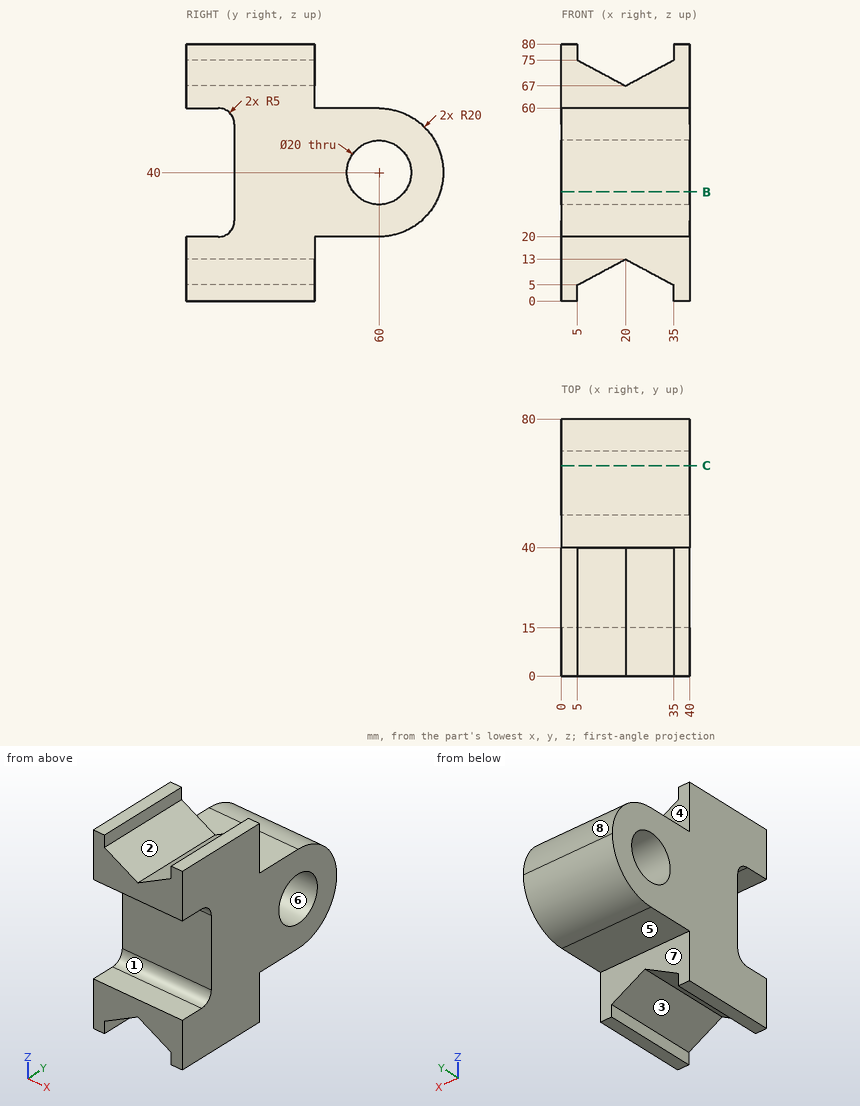
Input: dimensioned drawing with shaded views. Units: mm. Origin: part minimum x, y, z. A direction names the side the tool comes from. Round coordinates to 2 decimals unless told otherwise and drop trailing zeros. Order: outer loops, then holes, each group sorted by start corner. A loop starts at its lowest first (then second) coordinate and runs counter-clockwise, first axis right, second up. Notation, with made-up numbers: (73, 35.25) -> (102, 35.25) arc R15 cw to (102, 42.25) -> close; hole circle Ø2 at (-9, -13.5). An arc over 180 degrees is marked (long way). Put each result on its own line as item: value. Start each with the question number.
Q1. Section C-C on y = 65.5. Return the cut outline in (x, z).
Q2. First-contact query: pin 1 (6 mm diameter, centred on x = 12.5, y = 50.5, fed in from +Z); pin 2 (10 mm diameter, centred on x = 11, z = 70, fed in from +Y); pin 3 (22 mm diameter, centred on x = 16.5, z = 12, fed in from +Y). Flat tips, straight axial feed; report the tip coordinate or a pass-through.
Q3. Line query: probe 1 along Z at (x, y) = (13, 60); probe 2 along Y at (x, z) = (10, 40); probe 3 along Z at (x, y) = (2, 8.5). Output: solid intervals per line, ascending.
Q4. Section B-B on z = 34. Return the cut outline in (x, y).
Q5. Reachability of the marked faces 1, 2, 3, 4 and 5 from +Z, -Z, +X, -X, +Y, -Y: full face, straight path, thin tool, end or side. Return the list, or none.
Q6. Pull-direction query (Z, two-part tool) for the marked faces 6, 7 and 8; classes: +Z half, -Z half, draft (parallel to the pull), parting line (faces both ways), or undercut.
Ans:
1. outline: (0, 20.77) -> (40, 20.77) -> (40, 31.65) -> (0, 31.65) -> close; (0, 48.35) -> (40, 48.35) -> (40, 59.23) -> (0, 59.23) -> close
2. pin 1: stops at z = 60
2. pin 2: stops at y = 40
2. pin 3: stops at y = 70.54
3. probe 1: z = 20 to 30, 50 to 60
3. probe 2: y = 15 to 50, 70 to 80
3. probe 3: z = 0 to 20, 60 to 80
4. outline: (0, 15) -> (40, 15) -> (40, 52) -> (0, 52) -> close; (0, 68) -> (40, 68) -> (40, 79.08) -> (0, 79.08) -> close
5. face 1: +X, -X, -Y
5. face 2: +Z, +Y, -Y
5. face 3: -Z, +Y, -Y
5. face 4: +Z, +X, -X, +Y
5. face 5: -Z, +X, -X, +Y
6. face 6: undercut
6. face 7: draft
6. face 8: +Z half
